Autodesk Inventor part; units mm, degrees
ref_plane "YZ Plane" through (0, 0, 0) normal (1, 0, 0) x (0, 1, 0)
ref_plane "XZ Plane" through (0, 0, 0) normal (0, 1, 0) x (-1, 0, 0)
ref_plane "XY Plane" through (0, 0, 0) normal (0, 0, 1) x (1, 0, 0)
sketch "Szkic1" plane through (0, 0, 0) normal (1, 0, 0) x (0, 1, 0)
  line L0 (0, 0) -> (0, -88)
  line L1 (51.058, -70.4193) -> (51.058, -71.4193)
  line L2 (0, -88) -> (0, -97)
  line L3 (0, -97) -> (0, -98)
  line L4 (0, -98) -> (51.058, -80.4193)
  line L5 (51.058, -80.4193) -> (51.058, -79.4193)
  line L6 (51.058, -79.4193) -> (0, -97)
  line L7 (0, 0) -> (0, 1)
  line L8 (0, 1) -> (51.058, 1)
  line L9 (51.058, 1) -> (51.058, 2)
  line L10 (51.058, 2) -> (0, 2)
  line L11 (0, 2) -> (0, 1)
  dimension "d0" = 88
  dimension "d1" = 54
  dimension "d5" = 9
  dimension "d6" = 1
  dimension "d7" = 54
  dimension "d8" = 71
  dimension "d9" = 1
  dimension "d10" = 1
  dimension "d11" = 1
extrude "Wyciągnięcie proste1" add sketch "Szkic1" against normal blind 100
sketch "Szkic2" plane through (-100, 0, 0) normal (-1, 0, 0) x (0, 0, 1)
  line L0 (0, 10) -> (1, 10)
  line L1 (1, 51.058) -> (1, 0)
  line L2 (0, 10) -> (-93.5567, 10)
  line L3 (-79.4193, 51.058) -> (-97, 0)
  line L4 (0, 9) -> (1, 9)
  line L5 (0, 9) -> (-93.9011, 9)
  line L6 (-93.5567, 10) -> (-93.9011, 9)
  line L7 (1, 10) -> (1, 9)
  point P0 (0, 0)
  dimension "d14" = 10
  dimension "d15" = 1
extrude "Wyciągnięcie proste2" add sketch "Szkic2" against normal blind 100
sketch "Szkic3" plane through (-100, 51.058, -79.4193) normal (0, -0.3256, 0.9455) x (1, 0, 0)
  point P0 (100, -22.4199)
sketch "Szkic4" plane through (-100, 51.058, -80.4193) normal (0, 1, 0) x (1, 0, 0)
  line L0 (100, -81.4193) -> (100, 13.4817)
  line L1 (100, 0) -> (100, -1)
  line L2 (100, -81.4193) -> (100, -1)
  line L3 (0, -1) -> (0, 0)
  line L4 (100, -1) -> (0, -1)
  line L5 (0, 13.4817) -> (0, -81.4193)
  line L6 (0, -1) -> (0, -81.4193)
  line L7 (100, -81.4193) -> (0, -81.4193)
  line L8 (0, -81.4193) -> (100, -81.4193)
  point P0 (100, -80.4193)
extrude "Wyciągnięcie proste3" add sketch "Szkic4" against normal blind 1
sketch "Szkic5" plane through (-100, 9, -93.9011) normal (0, -1, 0) x (1, 0, 0)
  point P0 (100, 93.9011)
sketch "Szkic6" plane through (-100, 51.058, -79.4193) normal (-1, 0, 0) x (0, 0, -1)
  point P0 (-79.4193, 51.058)
sketch "Szkic7" plane through (-100, 9, -93.9011) normal (0, -1, 0) x (1, 0, 0)
  line L0 (100, 14.4817) -> (100, 94.9011)
  line L1 (100, 94.9011) -> (90, 94.9011)
  line L2 (0, 94.9011) -> (100, 94.9011)
  line L3 (90, 94.9011) -> (90, 0)
  line L4 (100, 0) -> (0, 0)
  line L5 (90, 0) -> (100, 0)
  line L6 (100, 0) -> (100, 94.9011)
  line L7 (90, 94.9011) -> (100, 94.9011)
  line L8 (0, 94.9011) -> (10, 94.9011)
  line L9 (10, 94.9011) -> (10, 0)
  line L10 (0, 0) -> (0, 94.9011)
  line L11 (10, 0) -> (0, 0)
  line L12 (0, 94.9011) -> (0, 14.4817)
  line L13 (0, 0) -> (0, 94.9011)
  line L14 (0, 94.9011) -> (10, 94.9011)
  point P0 (100, 93.9011)
  dimension "d20" = 10
  dimension "d21" = 10
extrude "Wyciągnięcie proste4" cut sketch "Szkic7" against normal blind 1 contours L6 L4 L3 L1 L0 | L9 L4 L10 L2
sketch "Szkic8" plane through (-90, 9, 1) normal (0, -1, 0) x (1, 0, 0)
  line L0 (80, -94.9011) -> (80, 0)
  line L1 (80, 0) -> (73, 0)
  line L2 (80, 0) -> (0, 0)
  line L3 (73, 0) -> (73, -94.9011)
  line L4 (80, -94.9011) -> (0, -94.9011)
  line L5 (80, -94.9011) -> (80, 0)
  line L6 (90, 1) -> (-10, 1)
  line L7 (80, 0) -> (73, 0)
  line L8 (0, 0) -> (7, 0)
  line L9 (7, 0) -> (7, -94.9011)
  line L10 (0, -94.9011) -> (7, -94.9011)
  line L11 (0, 0) -> (0, -94.9011)
  line L12 (0, -94.9011) -> (0, 0)
  line L13 (0, -94.5567) -> (0, 0)
  point P0 (90, -1)
  dimension "d24" = 7
  dimension "d25" = 7
extrude "Wyciągnięcie proste5" cut sketch "Szkic8" against normal blind 1 contours L4 L3 L1 L0 | L4 L11 L2 L9
sketch "Szkic9" plane through (-83, 9, -93.9011) normal (-1, 0, 0) x (0, 0, 1)
  line L0 (0, 0) -> (94.9011, 0)
  line L1 (0, 0) -> (5, 0)
  line L2 (5, 0) -> (1.9955, 3.0045)
  line L3 (5, 0) -> (9.2489, 0) construction
  line L4 (1.9955, 3.0045) -> (1.2807, 3.7193)
  line L5 (1.2807, 3.7193) -> (2.9085, 8.4469)
  line L6 (14.4817, 42.058) -> (0.3443, 1)
  line L7 (2.9085, 8.4469) -> (3.854, 8.1214)
  line L8 (3.854, 8.1214) -> (2.3383, 3.7193)
  line L9 (2.3383, 3.7193) -> (5, 1)
  line L10 (94.9011, 1) -> (0.3443, 1)
  line L11 (5, 1) -> (5, 0)
  point P0 (93.9011, -9)
  dimension "d28" = 5
  dimension "d29" = 135
  dimension "d31" = 5
  dimension "d32" = 1
extrude "Wyciągnięcie proste6" add sketch "Szkic9" against normal blind 66 contours L10 L6 L4 L2 | L2 L4 L5 L7 L8 L9 L10
sketch "Szkic10" plane through (-83, 12.7193, -91.5628) normal (0, -0.3256, 0.9455) x (1, 0, 0)
  line L0 (0.2651, 0) -> (15.2651, 0)
  line L1 (0, 0) -> (66, 0)
  line L2 (15.2651, 0) -> (15.2651, 2)
  line L3 (0, 4.6557) -> (66, 4.6557)
  circle A0 centre (15.2651, 2) radius 1.5
  line L4 (66, 0) -> (51, 0)
  line L5 (51, 0) -> (51, 2)
  circle A1 centre (51, 2) radius 1.5
  point P0 (83, 17.7836)
  dimension "d35" = 15
  dimension "d36" = 2
  dimension "d37" = 3
  dimension "d38" = 15
  dimension "d39" = 2
  dimension "d40" = 3
extrude "Wyciągnięcie proste7" cut sketch "Szkic10" against normal blind 15
sketch "Szkic11" plane through (-83, 9, -93.9011) normal (-1, 0, 0) x (0, 0, 1)
  line L0 (94.9011, 1) -> (5, 1)
  line L1 (94.9011, 1) -> (90.2011, 1)
  line L2 (90.2011, 1) -> (93.0515, 3.8505)
  line L3 (93.0515, 3.8505) -> (94.9011, 5.7)
  line L4 (94.9011, 41.058) -> (94.9011, -9)
  line L5 (90.2011, 1) -> (89.2011, 1)
  line L6 (94.9011, 0) -> (94.9011, 1)
  line L7 (94.9011, 1) -> (94.9011, 9)
  line L8 (94.9011, 9) -> (93.9011, 9)
  line L9 (93.9011, 9) -> (93.9011, 5.7)
  line L10 (93.9011, 5.7) -> (89.2011, 1)
  line L11 (94.9011, 9) -> (94.9011, 5.7)
  point P0 (93.9011, -9)
  dimension "d43" = 4.7
  dimension "d44" = 45
  dimension "d45" = 1
  dimension "d46" = 8
  dimension "d47" = 1
extrude "Wyciągnięcie proste8" add sketch "Szkic11" against normal blind 66
sketch "Szkic12" plane through (-83, 14.7, 0) normal (0, 0, -1) x (-1, 0, 0)
  point P0 (-83, -14.7)
sketch "Szkic13" plane through (-83, 9, -93.9011) normal (-1, 0, 0) x (0, 0, 1)
  line L0 (93.9011, 5.7) -> (89.2011, 1)
  line L1 (89.2011, 1) -> (91.885, 2.5496)
  line L2 (89.2011, 1) -> (92.3002, 1) construction
  line L3 (91.885, 2.5496) -> (93.9011, 3.7135)
  line L4 (93.9011, 5.7) -> (93.9011, 3.7135)
  line L5 (5, 1) -> (89.2011, 1)
  line L6 (93.9011, 5.7) -> (89.2011, 1)
  point P0 (93.9011, -9)
  dimension "d50" = 30
extrude "Wyciągnięcie proste9" cut sketch "Szkic13" against normal blind 66
sketch "Szkic14" plane through (-17, 18, 0) normal (0, 0, -1) x (-1, 0, 0)
  line L0 (66, -5.2865) -> (0, -5.2865)
  line L1 (66, -5.2865) -> (51, -5.2865)
  line L2 (51, -5.2865) -> (51, -3.2865)
  circle A0 centre (51, -3.2865) radius 1.5
  line L3 (0, -5.2865) -> (0, 0)
  line L4 (0, -5.2865) -> (15, -5.2865)
  line L5 (15, -5.2865) -> (15, -3.2865)
  circle A1 centre (15, -3.2865) radius 1.5
  point P0 (-17, -18)
  dimension "d53" = 15
  dimension "d54" = 2
  dimension "d55" = 3
  dimension "d56" = 15
  dimension "d57" = 2
  dimension "d58" = 3
extrude "Wyciągnięcie proste10" cut sketch "Szkic14" against normal blind 15
sketch "Szkic15" plane through (-83, 9, -93.9011) normal (-1, 0, 0) x (0, 0, 1)
  point P0 (93.9011, -9)
sketch "Szkic16" plane through (-17, 18, 0) normal (0, 0, -1) x (-1, 0, 0)
  point P0 (-17, -18)
sketch "Szkic17" plane through (-83, 9, -93.9011) normal (-1, 0, 0) x (0, 0, 1)
  line L0 (94.9011, 9) -> (93.9011, 9)
  line L1 (94.9011, 9) -> (94.9011, 8)
  line L2 (94.9011, 41.058) -> (94.9011, -9)
  line L3 (94.9011, 8) -> (93.9011, 8)
  line L4 (93.9011, 3.7135) -> (93.9011, 9)
  line L5 (93.9011, 9) -> (94.9011, 9)
  point P0 (93.9011, -9)
  dimension "d61" = 1
extrude "Wyciągnięcie proste11" cut sketch "Szkic17" against normal blind 66
properties part number "zderzaki"
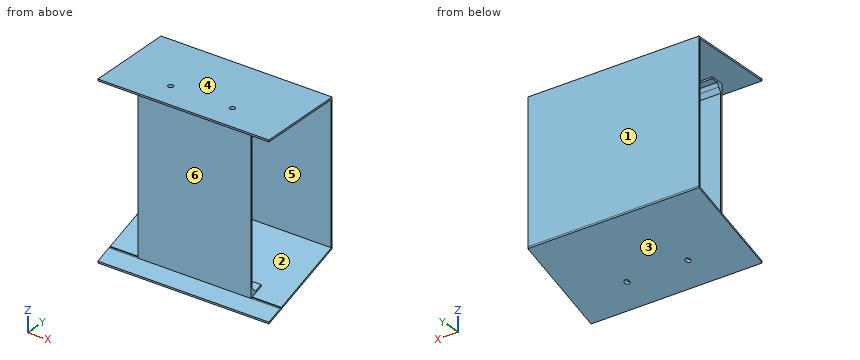
Check sheet for the modelled part. Datum: model origin and axes. Units: mm. Face numbers are marked on the shaded views. A direction names the side the tool comes from. Round coordinates to 2 decimals unless told otherwise and drop trailing zeros. Loops run counter-clockwise (first coordinate to the right, second up) from the corner with the lowest first, then second, coordinate; pieces in that order, holes last. Notation, with made-up numbers: (17, -3.75) - (70, -3.75) arc R16 ccw to (70, 7.25) - close; hole circle Ø5 at (-39, -3). An arc over 180 degrees is marked (long way). Write item = value, one per line. Start each with the question number.
Q1. Thickness scan on L1, parallel to Y at x = -68, z = 0.7; L2, parallel to Y at x = -30.5, z = -49.5; L3, parallel to Y at x = -5, z = -9. Record the ranges inside material, lowest first.
Q2. Access from +Z, -Z, +X, -X, +Y, -Y to the whole of each face (thin tool, end or side, straight path). Record for the marked faces 5 and 6.
Q3. Section check A-A (z = -46.5). Record the boundary of the cut face in (x, y).
Q4. Depth check by flat-ended pin: P1, Ø4, axis at x = -37.5, y = 29, coming from the -Z side; P2, Ø4.5, axis at x = -34.5, y = 15, coming from the -Z side; P3, Ø7, axis at y = 11, z = -62.5, coming from the +X side. Enter the tip coordinate at first touch or a pass-through.
Q5. Section check C-C (y = 28.5). Record the boundary of the cut face in (x, z).
Q6. Release check for a two-part mould opening along Z. For the marked faces 1, 2, 3 and 4 record: pulls with the +Z half, pulls with the -Z half, needs draft (parallel to the pull), parting line crosses it, or undercut.
Derived:
q1.L1 = 9 to 13.21, 16.21 to 17, 50.06 to 51.06
q1.L2 = 9 to 10, 50.06 to 51.06
q1.L3 = 50.06 to 51.06
q2.face_5 = +X, -X
q2.face_6 = +X, -X, -Y
q3.outline = (-100, 50.06) - (0, 50.06) - (0, 51.06) - (-100, 51.06) - close; (-83, 9) - (-17, 9) - (-17, 10) - (-83, 10) - close
q4.P1 = -88.7
q4.P2 = -93.61
q4.P3 = -17
q5.outline = (-100, -88.19) - (0, -88.19) - (0, -87.19) - (-100, -87.19) - close; (-100, 1) - (0, 1) - (0, 2) - (-100, 2) - close
q6.face_1 = needs draft
q6.face_2 = undercut
q6.face_3 = pulls with the -Z half
q6.face_4 = pulls with the +Z half
